Solid Edge part; units mm, degrees
sketch "Sketch1" plane through (0, 0, 0) normal (0, 0, 1) x (1, 0, 0)
  arc A0 (70, 100) -> (80, 90) centre (70, 90) cw
  line L0 (80, 90) -> (80, 10)
  arc A1 (80, 10) -> (70, 0) centre (70, 10) cw
  line L1 (70, 0) -> (0, 0)
  line L2 (0, 0) -> (0, 100)
  line L3 (0, 100) -> (70, 100)
  circle A2 centre (50, 50) radius 17.5
extrude "Protrusion1" add sketch "Sketch1" along normal blind 4
properties material "Acrílico, alto impacto"
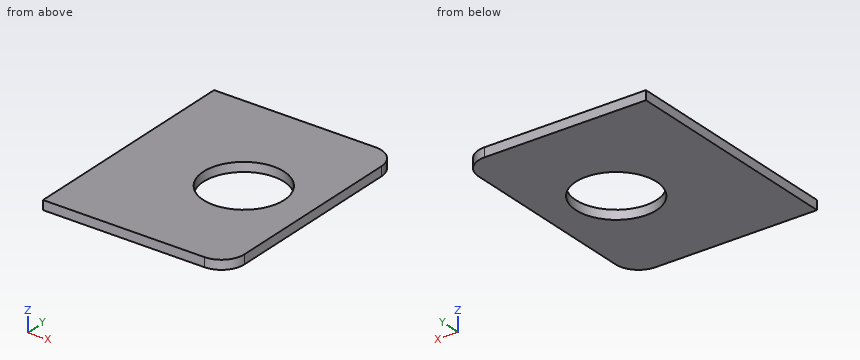
The model under review builds one solid part; all positions refer to its coordinate system, in mm. Round coordinates to 2 decimals unless told otherwise and drop trailing zeros. Order: outer loops, then holes, each group sorted by start corner. A loop starts at its lowest first (then second) coordinate and runs counter-clockwise, first axis right, second up.
(1) Take a section at A-A, the plane x = 50. State the section outline as (y, z) points, plus the area to 3 significant figures.
Working result:
outline: (0, 0) - (32.5, 0) - (32.5, 4) - (0, 4) - close; (67.5, 0) - (100, 0) - (100, 4) - (67.5, 4) - close
area: 260 mm2
(2) Take a section at D-D, the plane x = 75.5. State the section outline as (y, z) points.
Working result:
outline: (1.65, 0) - (98.35, 0) - (98.35, 4) - (1.65, 4) - close
(3) Wall thickness on L1, parallel to X at y = 49.5, z = 1.2; L2, parallel to Y at x = 50, z = 1.45; L3, parallel to X at y = 36, z = 2.9: over which ranges is each line inside the solid? List them lowest first.
Working result:
L1: x = 0 to 32.51, 67.49 to 80
L2: y = 0 to 32.5, 67.5 to 100
L3: x = 0 to 39.5, 60.5 to 80
(4) Take a section at C-C, the plane z = 1.15. State the section outline as (x, y) points.
Working result:
outline: (0, 0) - (70, 0) arc R10 ccw to (80, 10) - (80, 90) arc R10 ccw to (70, 100) - (0, 100) - close; hole circle Ø35 at (50, 50)
(5) Take a section at B-B, the plane y = 50. State the section outline as (x, z) points, plus the area to 3 significant figures.
Working result:
outline: (0, 0) - (32.5, 0) - (32.5, 4) - (0, 4) - close; (67.5, 0) - (80, 0) - (80, 4) - (67.5, 4) - close
area: 180 mm2
